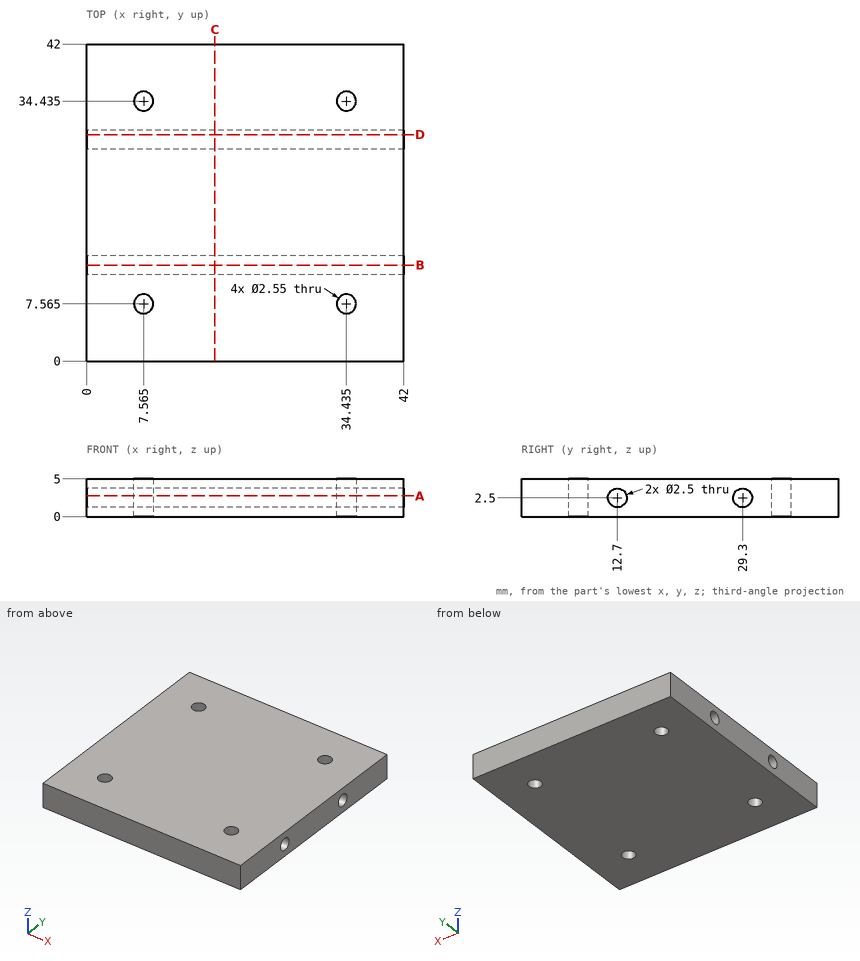
Part print with two shaded views. Sizes in mm from the minimum x, y, z corner. Coordinates: 2 decimals unless noted, no trailing zeros. Write each loop counter-clockwise with the first axis right and the second up, starting at its lowest first coordinate (ties: lowest second). Pieces come first, ordered by that corner, then holes. Notation, with made-up numbers: (8.25, -5.75) - (63.25, -5.75) arc R28 cw to (63.25, 19.25) - close; hole circle Ø10 at (79, 37). An arc over 180 degrees is marked (long way). Put each result on its own line as item: value.
1. Band-saw the part on B-B (y = 12.7). Write the cut outline in (x, z), then the cut area to 3 significant figures.
Final values:
outline: (0, 0) - (42, 0) - (42, 1.25) - (0, 1.25) - close; (0, 3.75) - (42, 3.75) - (42, 5) - (0, 5) - close
area: 105 mm²
2. Probe line 1 along Y through (x, z) = (27.5, 2.5); line 2 along X through (y, z) = (34.5, 0.35); line 3 along X through (y, z) = (6.5, 3.5). List the from-to ranges inside material, lowest first. Write a range as [from, to].
Final values:
line 1: y = [0, 11.45], [13.95, 28.05], [30.55, 42]
line 2: x = [0, 6.29], [8.84, 33.16], [35.71, 42]
line 3: x = [0, 6.86], [8.27, 33.73], [35.14, 42]
3. Band-saw the part on D-D (y = 30). Write the cut outline in (x, z).
Final values:
outline: (0, 0) - (42, 0) - (42, 1.46) - (0, 1.46) - close; (0, 3.54) - (42, 3.54) - (42, 5) - (0, 5) - close
4. Flat gauge pins, fed straight in: pin 1 Ø4 at (x, y) = (34.44, 7.56) entering from -Z; pin 2 Ø1.5 at (x, y) = (7.56, 34.44) entering from +Z. Where does each tip first touch, or does it go through?
Final values:
pin 1: stops at z = 0
pin 2: passes through
5. Band-saw the part on C-C (x = 17). Write the cut outline in (y, z).
Final values:
outline: (0, 0) - (42, 0) - (42, 5) - (0, 5) - close; hole circle Ø2.5 at (12.7, 2.5); hole circle Ø2.5 at (29.3, 2.5)
6. Band-saw the part on A-A (z = 2.75). Write the cut outline in (x, y) (3 decimals).
Final values:
outline: (0, 0) - (42, 0) - (42, 11.475) - (0, 11.475) - close; (0, 13.925) - (42, 13.925) - (42, 28.075) - (0, 28.075) - close; (0, 30.525) - (42, 30.525) - (42, 42) - (0, 42) - close; hole circle Ø2.55 at (7.565, 7.565); hole circle Ø2.55 at (7.565, 34.435); hole circle Ø2.55 at (34.435, 7.565); hole circle Ø2.55 at (34.435, 34.435)
